Work out the finished part from the listing and answer in its coordinate system (mm). A direction names the side the tool comes from. Round coordinates to 2 decimals unless told otherwise and drop trailing zeros. Write each loop counter-clockwise with the first axis right and the second up, starting at its lowest first coordinate (ties: lowest second). Pieces come first, ordered by that corner, then holes. Notation, with made-up numbers: (-10, -13.75) -> (1, -13.75) arc R23 cw to (1, 16.25) -> close; hole circle Ø8 at (8, 75.25). An arc over 180 degrees is marked (long way). One line per item, written item: value.
```python
from build123d import *

# Parameters (mm, degrees)
SKETCH_1_W         = 31
SKETCH_1_H         = 54
SKETCH_1_W_2       = 21
SKETCH_1_H_2       = 41
EXTRUDE_1_DEPTH    = 5
SKETCH_2_W         = 5
SKETCH_2_H         = 10
EXTRUDE_2_DEPTH    = 7.5
HOLE_WIZARD_M3_1_D = 2.5


with BuildPart() as part:
    # 草图1 → 凸台-拉伸1 (new body)
    with BuildSketch(Plane.XY):
        Rectangle(SKETCH_1_W, SKETCH_1_H)
        Rectangle(SKETCH_1_W_2, SKETCH_1_H_2, mode=Mode.SUBTRACT)
    extrude(amount=EXTRUDE_1_DEPTH)

    # 草图2 → 凸台-拉伸2 (add)
    with BuildSketch(Plane(origin=(15.5, 0, 0), x_dir=(0, 0, -1), z_dir=(1, 0, 0))):
        with Locations((-2.5, 9.2)):
            Rectangle(SKETCH_2_W, SKETCH_2_H)
    extrude_2 = extrude(amount=EXTRUDE_2_DEPTH)

    # 镜向1: 凸台-拉伸2 across plane
    add(extrude_2.mirror(Plane(origin=(0, 0, 0), x_dir=(0, 0, 1), z_dir=(1, 0, 0))))

    # M3 螺纹孔1 (through all)
    with Locations(Plane(origin=(0, 0, 0), x_dir=(-1, 0, 0), z_dir=(0, 0, -1))):
        with Locations((-5, -24), (5, -24), (-5, 24), (5, 24)):
            Hole(HOLE_WIZARD_M3_1_D / 2)

    # 草图7 → M3 螺纹孔2 (revolve, cut)
    with BuildSketch(Plane(origin=(23, 9.2, 2.5), x_dir=(0, 0, -1), z_dir=(0, 1, 0))):
        Polygon((0, 0), (0, 6.251075774), (1.25, 5.5), (1.25, 0), align=None)
    hole_wizard_m3_2 = revolve(axis=Axis((29.35, 9.2, 2.5), (-1, 0, 0)), mode=Mode.SUBTRACT)

    # 镜向2: M3 螺纹孔2 across plane
    add(hole_wizard_m3_2.mirror(Plane(origin=(0, 0, 0), x_dir=(0, 0, 1), z_dir=(1, 0, 0))), mode=Mode.SUBTRACT)


solid = part.part
```
(1) Find section B-B on y = 0. Give the vertices of the cut face in (x, z).
Reported:
outline: (-15.5, 0) -> (-10.5, 0) -> (-10.5, 5) -> (-15.5, 5) -> close; (10.5, 0) -> (15.5, 0) -> (15.5, 5) -> (10.5, 5) -> close
(2) Find section A-A on y = -24. Give the vertices of the cut face in (x, z).
Reported:
outline: (-15.5, 0) -> (-6.25, 0) -> (-6.25, 5) -> (-15.5, 5) -> close; (-3.75, 0) -> (3.75, 0) -> (3.75, 5) -> (-3.75, 5) -> close; (6.25, 0) -> (15.5, 0) -> (15.5, 5) -> (6.25, 5) -> close
(3) Find section C-C on x = -5. Give the vertices of the cut face in (y, z), plus the area to 3 significant figures.
Reported:
outline: (-27, 0) -> (-25.25, 0) -> (-25.25, 5) -> (-27, 5) -> close; (-22.75, 0) -> (-20.5, 0) -> (-20.5, 5) -> (-22.75, 5) -> close; (20.5, 0) -> (22.75, 0) -> (22.75, 5) -> (20.5, 5) -> close; (25.25, 0) -> (27, 0) -> (27, 5) -> (25.25, 5) -> close
area: 40.0 mm2
(4) A tool of negligible diameter and unlimited length cuts with its end or side. For faces 1 (the face through (-15.5, 21, 2)), 2 (the face through (20.288, 8.146, 1.828)), 3 (the face through (-19, 4.2, 3)), 4 (the face through (15.5, 21, 2)), from which of +Z, -Z, +X, -X, +Y, -Y can it reach the whole face along a straight path? Write none if from no direction.
Reported:
face 1: +Z, -Z, -X, +Y
face 2: +X
face 3: +Z, -Z, -X, -Y
face 4: +Z, -Z, +X, +Y
(5) Flat-ended cylindrical pins translate along their axes: pin 1 Ø2.5 at (y, z) = (18, 3) entering from +X; pin 2 Ø2.5 at (x, z) = (-18, 2) entering from -Y; pin 3 Ø2.5 at (x, z) = (-18, 2.5) entering from +Y. Find the tip coordinate at first contact, or state that the pin passes through.
Reported:
pin 1: stops at x = 15.5
pin 2: stops at y = 4.2
pin 3: stops at y = 14.2
(6) Consider probe 1 along Y at (x, z) = (-5, 3.8); probe 2 along X at (y, z) = (-12, 2.2); probe 3 along Z at (x, y) = (-19.9, 9.2). Determine where each line is inside the solid, lowest interval first.
Reported:
probe 1: y = -27 to -25.25, -22.75 to -20.5, 20.5 to 22.75, 25.25 to 27
probe 2: x = -15.5 to -10.5, 10.5 to 15.5
probe 3: z = 0 to 1.25, 3.75 to 5
(7) For a pull along X with two mould halves and no side action, classify faces 5 (the face through (0, -20.5, 2)), 6 (the face through (0, -27, 2)), 7 (the face through (15.5, -12, 2)) as pulls with the +X half, pulls with the -X half, needs draft (parallel to the pull), parting line crosses it, or undercut.
Reported:
face 5: undercut
face 6: needs draft
face 7: pulls with the +X half
